Part print with two shaded views. Sizes in mm from the minimum x, y, z corner. Give positions to 0.01 mm unless a question says otherwise; leave off trailing zeros. Write each loop counter-clockwise with the first axis right and the second up, starting at its lowest first coordinate (ties: lowest second). Pieces come first, ordered by that corner, then holes. Notation, with made-up numbers: (55.25, -39.75) - (83.25, -39.75) arc R23 cw to (83.25, -17.75) - close; hole circle Ø1 at (19, 24). An arc over 180 degrees is marked (long way). One line per item, written item: value. Start each with the question number.
(1) Drop flat-ended pins along their axis: P1, Ø5, axis at y = 9.5, z = 99, coming from the -X side; P2, Ø1.5, axis at x = 171, z = 64.5, coming from the -Y side; P3, Ø6.5, axis at x = 61, y = 4.5, coming from the -Z side; P4, Ø8.5, axis at x = 25.4, z = 187.325, coming from the -Y side. Give the stop position or say it passes through.
(2) Cut at C-C, the plane y = 10. State how many separate pieces and enclosed holes the cut face has, and give its area (3 significant figures).
(3) Probe L1, parallel to Z at x = 279.4, y = 9.75; L2, parallel to Z at x = 276, y = 0.5; L3, parallel to X at y = 8.5, z = 45. List the from-to ranges inside material, lowest first.
(4) Cut at B-B, the plane z = 25.4. List the corners of the cut face in (x, y).
(5) Cut at A-A, the plane x = 25.4. List the corners of the cut face in (y, z), and give its area (3 significant figures).
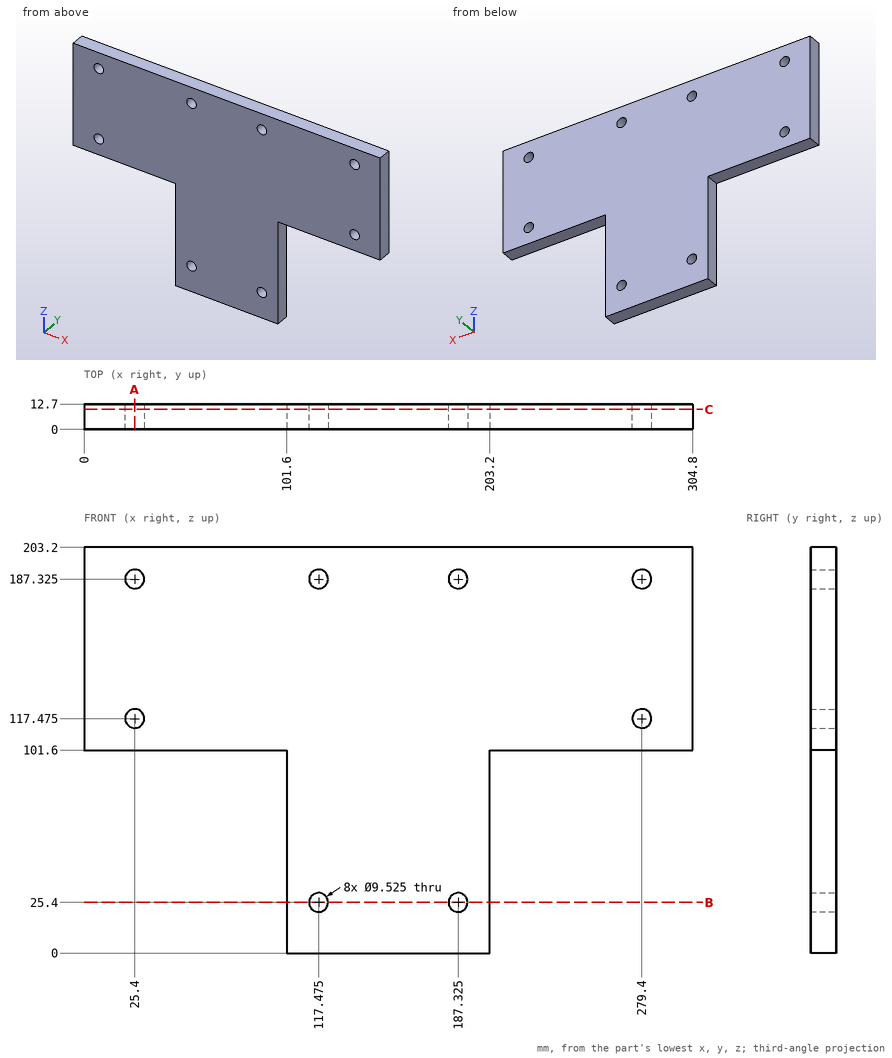
Answers follow:
1. P1: stops at x = 101.6
1. P2: stops at y = 0
1. P3: stops at z = 101.6
1. P4: passes through
2. separate pieces: 1
2. enclosed holes: 8
2. area: 40,700 mm²
3. L1: z = 101.6 to 112.71, 122.24 to 182.56, 192.09 to 203.2
3. L2: z = 101.6 to 114.14, 120.81 to 183.99, 190.66 to 203.2
3. L3: x = 101.6 to 203.2
4. outline: (101.6, 0) - (112.71, 0) - (112.71, 12.7) - (101.6, 12.7) - close; (122.24, 0) - (182.56, 0) - (182.56, 12.7) - (122.24, 12.7) - close; (192.09, 0) - (203.2, 0) - (203.2, 12.7) - (192.09, 12.7) - close
5. outline: (0, 101.6) - (12.7, 101.6) - (12.7, 112.71) - (0, 112.71) - close; (0, 122.24) - (12.7, 122.24) - (12.7, 182.56) - (0, 182.56) - close; (0, 192.09) - (12.7, 192.09) - (12.7, 203.2) - (0, 203.2) - close
5. area: 1,050 mm²
